from build123d import *

# Parameters (mm, degrees)
SKETCH1_R           = 5.08
SKETCH1_R_2         = 1.778
BOSS_EXTRUDE1_DEPTH = 10.16
SKETCH3_W           = 12.7
SKETCH3_H           = 12.7
BOSS_EXTRUDE2_DEPTH = 101.6
SKETCH6_W           = 7.62
SKETCH6_H           = 7.62
BOSS_EXTRUDE3_DEPTH = 6.35
BOSS_EXTRUDE4_START = -12.7
BOSS_EXTRUDE4_DEPTH = 12.7
FILLET2_R           = 2.54
BOSS_EXTRUDE5_START = -12.7
SKETCH7_W           = 57.15
SKETCH7_H           = 5.08
BOSS_EXTRUDE5_DEPTH = 12.7
SKETCH9_W           = 25.4
SKETCH9_H           = 25.4
CUT_EXTRUDE1_DEPTH  = 111.76
BOSS_EXTRUDE6_DEPTH = 12.7
FILLET3_R           = 2.54
SKETCH12_W          = 5.08
SKETCH12_H          = 30.48
BOSS_EXTRUDE7_DEPTH = 3.175
SKETCH13_W          = 7.874
SKETCH13_H          = 7.874
CUT_EXTRUDE3_DEPTH  = 6.35


with BuildPart() as part:
    # Sketch1 → Boss-Extrude1 (new body)
    with BuildSketch(Plane.XY):
        with BuildLine():
            Line((-6.35, 12.7), (-6.35, 10.998522628))
            ThreePointArc((-6.35, 10.998522628), (0, -12.7), (6.35, 10.998522628))
            Line((6.35, 10.998522628), (6.35, 43.18))
            Line((6.35, 43.18), (6.35, 93.98))
            Line((6.35, 93.98), (-6.35, 93.98))
            Line((-6.35, 93.98), (-6.35, 12.7))
        make_face()
        Circle(SKETCH1_R, mode=Mode.SUBTRACT)
        with Locations((0, 8.128)):
            Circle(SKETCH1_R_2, mode=Mode.SUBTRACT)
        with Locations((8.128, 0)):
            Circle(SKETCH1_R_2, mode=Mode.SUBTRACT)
        with Locations((0, -8.128)):
            Circle(SKETCH1_R_2, mode=Mode.SUBTRACT)
        with Locations((-8.128, 0)):
            Circle(SKETCH1_R_2, mode=Mode.SUBTRACT)
    extrude(amount=BOSS_EXTRUDE1_DEPTH)

    # Sketch3 → Boss-Extrude2 (add)
    with BuildSketch(Plane.XY.offset(10.16)):
        with Locations((0, 25.4)):
            Rectangle(SKETCH3_W, SKETCH3_H)
    extrude(amount=BOSS_EXTRUDE2_DEPTH)

    # Sketch6 → Boss-Extrude3 (add)
    with BuildSketch(Plane.XY.offset(111.76)):
        with Locations((0, 25.4)):
            Rectangle(SKETCH6_W, SKETCH6_H)
    extrude(amount=BOSS_EXTRUDE3_DEPTH)

    # Sketch5 → Boss-Extrude4 (add)
    with BuildSketch(Plane.ZY.offset(6.35).offset(BOSS_EXTRUDE4_START)):
        Polygon((31.75, 63.5), (60.96, 31.75), (54.057179058, 31.75), (49.383579058, 36.83), (29.520779058, 58.42), (10.16, 79.464325063), (10.16, 86.967391304), align=None)
    extrude(amount=BOSS_EXTRUDE4_DEPTH)

    # Fillet2
    fillet2_edges = [part.edges().sort_by_distance(p)[0] for p in [
        (0, 31.75, 60.96),
    ]]
    fillet(fillet2_edges, radius=FILLET2_R)

    # Sketch7 → Boss-Extrude5 (add)
    with BuildSketch(Plane(origin=(6.35, 0, 0), x_dir=(0, 0, -1), z_dir=(1, 0, 0)).offset(BOSS_EXTRUDE5_START)):
        with Locations((28.575, 91.44)):
            Rectangle(SKETCH7_W, SKETCH7_H)
    extrude(amount=BOSS_EXTRUDE5_DEPTH)

    # Sketch9 → Cut-Extrude1 (cut)
    with BuildSketch(Plane.XY.offset(111.76)):
        Rectangle(SKETCH9_W, SKETCH9_H)
    extrude(amount=-CUT_EXTRUDE1_DEPTH, mode=Mode.SUBTRACT)

    # Sketch11 → Boss-Extrude6 (add)
    with BuildSketch(Plane(origin=(6.35, 0, 0), x_dir=(0, 0, -1), z_dir=(1, 0, 0))):
        Polygon((0, 79.814999882), (57.15, 88.9), (0, 88.9), align=None)
    extrude(amount=-BOSS_EXTRUDE6_DEPTH)

    # Fillet3
    fillet3_edges = [part.edges().sort_by_distance(p)[0] for p in [
        (0, 79.814999882, 0),
        (0, 31.75, 10.16),
        (0, 19.05, 10.16),
        (0, 86.967391304, 10.16),
        (0, 79.464325063, 10.16),
        (0, 31.75, 54.057179058),
    ]]
    fillet(fillet3_edges, radius=FILLET3_R)

    # Sketch12 → Boss-Extrude7 (add)
    with BuildSketch(Plane(origin=(0, 93.98, 0), x_dir=(1, 0, 0), z_dir=(0, 1, 0))):
        with Locations((0, 34.29)):
            Rectangle(SKETCH12_W, SKETCH12_H)
    extrude(amount=BOSS_EXTRUDE7_DEPTH)

    # Sketch13 → Cut-Extrude3 (cut)
    with BuildSketch(Plane.XZ.offset(-12.7)):
        with Locations((0, 5.08)):
            Rectangle(SKETCH13_W, SKETCH13_H)
    extrude(amount=-CUT_EXTRUDE3_DEPTH, mode=Mode.SUBTRACT)


solid = part.part
Could you check a few things on this model? Use its own coordinates, in mm. A direction names the side the tool comes from. Round coordinates to 2 decimals unless told otherwise and drop trailing zeros. Write each loop counter-clockwise with the first axis right and the second up, starting at its lowest first coordinate (ties: lowest second). Pieces come first, ordered by that corner, then holes. Notation, with made-up numbers: (76, -7.75) - (101, -7.75) arc R34 ccw to (101, 28.25) - close; hole circle Ø11 at (49, 72.5). An arc over 180 degrees is marked (long way). Use a Markdown table: item, result.
Q1. I want a section at A-A (y = 60.5). List the corners of the cut face in (x, z) for me, plus the area to 3 significant figures.
Output values:
| item | result |
|---|---|
| outline | (-6.35, 0) - (6.35, 0) - (6.35, 10.16) - (-6.35, 10.16) - close; (-6.35, 27.61) - (6.35, 27.61) - (6.35, 34.51) - (-6.35, 34.51) - close |
| area | 217 mm2 |
Q2. I want a section at B-B (z = 5.5). List the corners of the cut face in (x, y) for me, plus the area to 3 significant figures.
Output values:
| item | result |
|---|---|
| outline | (-6.35, 12.7) - (-3.94, 12.7) - (-3.94, 19.05) - (3.94, 19.05) - (3.94, 12.7) - (6.35, 12.7) - (6.35, 93.98) - (-6.35, 93.98) - close |
| area | 982 mm2 |
Q3. I want a section at D-D (z = 53). List the corners of the cut face in (x, y) for me, plus the area to 3 significant figures.
Output values:
| item | result |
|---|---|
| outline | (-6.35, 19.05) - (6.35, 19.05) - (6.35, 40.4) - (-6.35, 40.4) - close |
| area | 271 mm2 |
Q4. I want a section at C-C (y = 24). List the corners of the cut face in (x, z) for me, plus the area to 3 significant figures.
Output values:
| item | result |
|---|---|
| outline | (-6.35, 0) - (6.35, 0) - (6.35, 111.76) - (3.81, 111.76) - (3.81, 118.11) - (-3.81, 118.11) - (-3.81, 111.76) - (-6.35, 111.76) - close |
| area | 1,470 mm2 |
Q5. For pin 1 (3 mm diameter, centred on y = 25.5, z = 114, fed in from -X); pin 2 (6.5 mm diameter, centred on x = 0.5, y = 60, fed in from -Z); pin 3 (1.9 mm diameter, centred on x = -1, z = 113.5, fed in from +Y), each with a flat end and sliding along its axis, tell me the tip position at first contact or that it passes through.
Output values:
| item | result |
|---|---|
| pin 1 | x = -3.81 |
| pin 2 | z = 0 |
| pin 3 | y = 29.21 |
Q6. Please list where these lines run through material, in increasing order: L1, parallel to Y at x = 2.25, z = 86; L2, parallel to Z at x = 1.5, y = 24; L3, parallel to Z at x = 1.5, y = 38.
Output values:
| item | result |
|---|---|
| L1 | 19.05 to 31.75 |
| L2 | 0 to 118.11 |
| L3 | 0 to 10.16, 48.31 to 55.21 |
Q7. For faces 1 (the flat face through (3.81, 25, 115)), 2 (the flat face through (0, 16, 1.143)), 3 (the flat face through (0, 15, 10.16)), which set-ups out of +Z, -Z, +X, -X, +Y, -Y let a thin tool reach every point of the face, with its end or its side?
Output values:
| item | result |
|---|---|
| face 1 | +Z, +X, +Y, -Y |
| face 2 | -Y |
| face 3 | +Z, +X, -X, -Y |
Q8. Thinking about a two-plate mould opening in X: for faces 4 (the cylindrical face through (-0.089, 75.333, 11.817)), 5 (the flat face through (-3.937, 16, 5)), 6 (the flat face through (6.35, 57, 34)), which applies, released by +X, released by -X, zero draft, split by the parting line, or undercut?
Output values:
| item | result |
|---|---|
| face 4 | zero draft |
| face 5 | undercut |
| face 6 | released by +X |
